Job drawing, mm, ordinate dimensions from the low corner. One solid piece. A direction names the side the tool comes from. Give positions to 0.01 mm unless a question says otherwise; leave off trailing zeros. Order: outer loops, then holes, each group sorted by start corner. A loop starts at its lowest first (then second) coordinate and runs counter-clockwise, first axis right, second up.
1. Slice it at C-C on y = 8. List the corners of the cut face in (x, z) (3 decimals).
2. Which spindle directions (+Z, -Z, +X, -X, +Y, -Y) get a long thin tool onto all of the face, cutting with end or side? Do the marked faces 5, 6, 7 and 8. Say none if no direction does.
3. Probe line 1 (X direction, y = 12.25, z = 6.5); line 2 (X direction, y = 12.5, z = 3.5); line 3 (Z direction, x = 78, y = 17.5). List the from-to ranges inside material, lowest first.
4. Mould opens along X. For the marked faces 1, 2, 3 and 4 say: +X half, -X half, draft (parallel to the pull), parting line (faces both ways), or undercut.
5. Drop flat-ended pins along their axis: pin 1 Ø2 at (y, z) = (10.5, 7) entering from +X; pin 2 Ø11 at (x, y) = (9, 9.5) entering from +Z; pin 3 Ø5.5 at (x, y) = (46, 12.5) entering from -Z; pin 4 Ø8 at (x, y) = (73.787, 9.525) entering from -Z. Give the stop position or say it passes through.
6. Slice it at A-A on z = 31. List the corners of the cut face in (x, y), and give its area (3 significant figures).
7. Slice it at B-B on y = 15.75. List the corners of the cut face in (x, z).
8. Slice it at D-D on x = 29. List the corners of the cut face in (y, z), and give its area (3 significant figures).
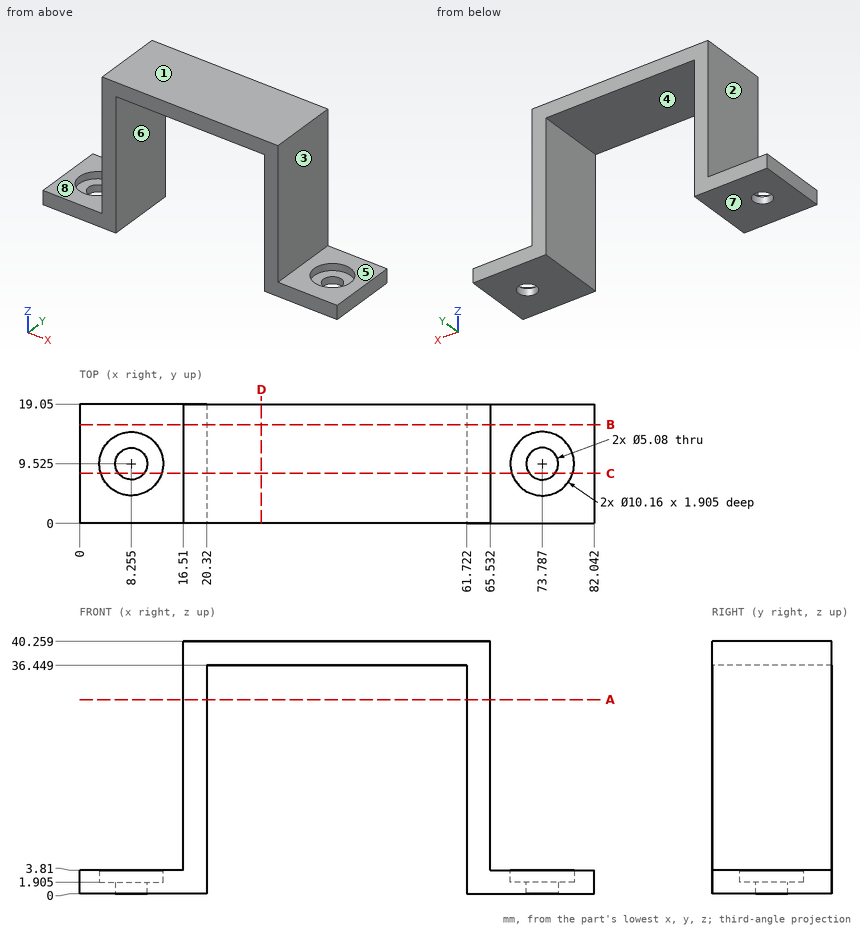
Data:
1. outline: (0, 0) - (6.224, 0) - (6.224, 1.905) - (3.409, 1.905) - (3.409, 3.81) - (0, 3.81) - close; (10.286, 0) - (20.32, 0) - (20.32, 36.449) - (61.722, 36.449) - (61.722, 0) - (71.756, 0) - (71.756, 1.905) - (68.941, 1.905) - (68.941, 3.81) - (65.532, 3.81) - (65.532, 40.259) - (16.51, 40.259) - (16.51, 3.81) - (13.101, 3.81) - (13.101, 1.905) - (10.286, 1.905) - close; (75.818, 0) - (82.042, 0) - (82.042, 3.81) - (78.633, 3.81) - (78.633, 1.905) - (75.818, 1.905) - close
2. face 5: +Z, +X, +Y, -Y
2. face 6: -Z, +Y, -Y
2. face 7: -Z, +X, -X, +Y, -Y
2. face 8: +Z, -X, +Y, -Y
3. line 1: x = 16.51 to 20.32, 61.72 to 65.53
3. line 2: x = 0 to 4.14, 12.37 to 20.32, 61.72 to 69.67, 77.9 to 82.04
3. line 3: z = 0 to 3.81
4. face 1: draft
4. face 2: -X half
4. face 3: +X half
4. face 4: undercut
5. pin 1: stops at x = 65.53
5. pin 2: stops at z = 3.81
5. pin 3: stops at z = 36.45
5. pin 4: stops at z = 0
6. outline: (16.51, 0) - (20.32, 0) - (20.32, 19.05) - (16.51, 19.05) - close; (61.72, 0) - (65.53, 0) - (65.53, 19.05) - (61.72, 19.05) - close
6. area: 145 mm2
7. outline: (0, 0) - (20.32, 0) - (20.32, 36.45) - (61.72, 36.45) - (61.72, 0) - (82.04, 0) - (82.04, 3.81) - (65.53, 3.81) - (65.53, 40.26) - (16.51, 40.26) - (16.51, 3.81) - (0, 3.81) - close
8. outline: (0, 36.45) - (19.05, 36.45) - (19.05, 40.26) - (0, 40.26) - close
8. area: 72.6 mm2
